Geometry check sheet. Reference: the model listing, model coordinates, mm. Face numbers are marked on the shaded views. A direction names the side the tool comes from. Give positions to 0.01 mm unless a question says otherwise; leave off trailing zeros. Write each loop counter-clockwise with the first axis right and the second up, starting at its lowest first coordinate (ties: lowest second). Pieces come first, ordered by that corner, then holes. Notation, with made-up numbers: (72, -28) - (92, -28) arc R13 cw to (92, -10) - close; hole circle Ø7 at (88.5, 2.25). An arc over 180 degrees is marked (long way). One line per question, with ' | ' between items. Start each with the question number.
Q1. Section check B-B on x = -52. Record the boundary of the cut face in (y, z), and give its area (3 significant figures).
Q2. Set-up check for the marked faces 4 and 5: record each of +Z, -Z, +X, -X, +Y, -Y from which the full face is reachable in a straight line by a thin tool's end or side.
Q3. Release check for a two-part mould opening along Z. For the marked faces 1, 2 and 3 record: +Z half, -Z half, draft (parallel to the pull), parting line (faces both ways), or undercut.
Q4. Section check D-D on y = 17. Record the boundary of the cut face in (x, z), and give its area (3 significant figures).
Q5. Thickness scan on L1, parallel to X at y = -54, z = 2.5; L2, parallel to Z at x = -17, y = 1; L3, parallel to Z at x = -24.5, y = -15. Record the ranges inside material, lowest first. Write a range as [from, to].
Q6. Section check C-C on x = -21.5. Record the boundary of the cut face in (y, z), and give its area (3 significant figures).
Q7. Gauge pin test, flat ends, axial feed: P1, Ø10, axis at x = -28, y = -16.5, coming from the +Z side; P2, Ø2, axis at x = -43, z = 7, coming from the -Y side. Record the tip position at first contact, or that the pin passes through.
Q8. Section check A-A on z = 2.5. Record the boundary of the cut face in (x, y).
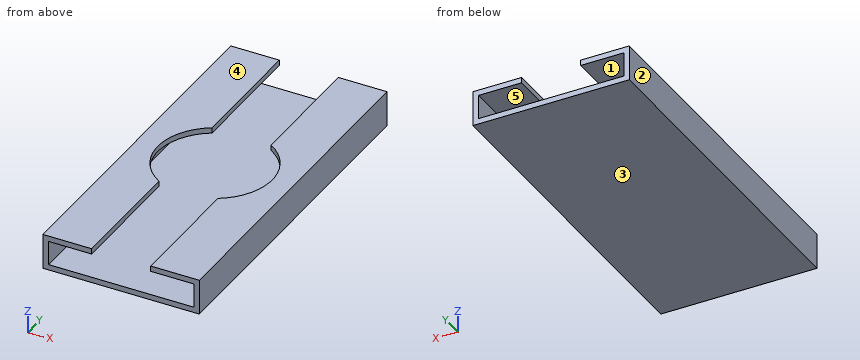
```python
from build123d import *

# Parameters (mm, degrees)
F0_W     = 45
F0_H     = 100
F1_DEPTH = 10.2
F2_W     = 17
F2_H     = 100
F3_DEPTH = 8.6
F4_W     = 41.8
F4_H     = 100
F5_DEPTH = 7
F8_R     = 16.5
F9_DEPTH = 10


with BuildPart() as f1:
    # F0 (on Top) → F1 (new body)
    with BuildSketch(Plane.XY):
        with Locations((-33.835356, -14.808846)):
            Rectangle(F0_W, F0_H)
    extrude(amount=F1_DEPTH)

    # F2 (on face) → F3 (cut)
    with BuildSketch(Plane.XY.offset(10.2)):
        with Locations((-33.835356, -14.808846)):
            Rectangle(F2_W, F2_H)
    extrude(amount=-F3_DEPTH, mode=Mode.SUBTRACT)


with BuildPart() as f5:
    # F4 (on Top) → F5 (new body)
    with BuildSketch(Plane.XY):
        with Locations((-35.435356, -14.808846)):
            Rectangle(F4_W, F4_H)
    extrude(amount=F5_DEPTH)


with BuildPart() as f5_1:
    # F6: moved
    add(f5.part.moved(Location((1.6, 0, 1.6))))


with BuildPart() as f1_1:
    add(f1.part)

    # F7: cut F5
    add(f5_1.part, mode=Mode.SUBTRACT)


with BuildPart() as f9:
    # F8 (on Top) → F9 (new body)
    with BuildSketch(Plane.XY):
        with Locations((-33.835356, -64.808846)):
            Circle(F8_R)
    extrude(amount=F9_DEPTH)


with BuildPart() as f9_1:
    # F10: moved
    add(f9.part.moved(Location((0, 50, 4))))


with BuildPart() as f1_2:
    add(f1_1.part)

    # F11: cut F9
    add(f9_1.part, mode=Mode.SUBTRACT)


solid = f1_2.part
```
Working result:
1) outline: (-64.81, 0) - (35.19, 0) - (35.19, 1.6) - (-64.81, 1.6) - close; (-64.81, 8.6) - (35.19, 8.6) - (35.19, 10.2) - (-64.81, 10.2) - close | area: 320 mm2
2) face 4: +Z, +X, -X, +Y, -Y | face 5: +Y, -Y
3) face 1: undercut | face 2: draft | face 3: -Z half
4) outline: (-56.34, 0) - (-11.34, 0) - (-11.34, 10.2) - (-25.34, 10.2) - (-25.34, 8.6) - (-12.94, 8.6) - (-12.94, 1.6) - (-54.74, 1.6) - (-54.74, 8.6) - (-42.34, 8.6) - (-42.34, 10.2) - (-56.34, 10.2) - close | area: 139 mm2
5) L1: x = [-56.34, -54.74], [-12.94, -11.34] | L2: z = [0, 1.6], [8.6, 10.2] | L3: z = [0, 1.6]
6) outline: (-64.81, 0) - (35.19, 0) - (35.19, 1.6) - (-64.81, 1.6) - close; (-64.81, 8.6) - (-25.77, 8.6) - (-25.77, 10.2) - (-64.81, 10.2) - close; (-3.85, 8.6) - (35.19, 8.6) - (35.19, 10.2) - (-3.85, 10.2) - close | area: 285 mm2
7) P1: stops at z = 1.6 | P2: passes through
8) outline: (-56.34, -64.81) - (-54.74, -64.81) - (-54.74, 35.19) - (-56.34, 35.19) - close; (-12.94, -64.81) - (-11.34, -64.81) - (-11.34, 35.19) - (-12.94, 35.19) - close
